Design review of the part built by this model. Coordinates are the model's own, in mm. A direction names the side the tool comes from. Coordinates: 2 decimals unless noted, no trailing zeros. Loops run counter-clockwise (first coordinate to the right, second up) from the corner with the lowest first, then second, coordinate; pieces in that order, holes last. Notation, with made-up numbers: (38, -27.75) - (78, -27.75) arc R31 ccw to (78, 2.25) - close; hole circle Ø3 at (-33, -33). An arc over 180 degrees is marked (long way). Return JSON: item names as keys, results as strings. Group by question number.
from build123d import *

# Parameters (mm, degrees)
SKETCH1_R           = 2.1
SKETCH1_R_2         = 1.6
SKETCH1_W           = 120
SKETCH1_H           = 56
SKETCH1_R_3         = 2.5
SKETCH1_R_4         = 3
BOSS_EXTRUDE1_DEPTH = 7
FILLET1_R           = 6


with BuildPart() as part:
    # Sketch1 → Boss-Extrude1 (new body)
    with BuildSketch(Plane(origin=(0, 0, 0), x_dir=(1, 0, 0), z_dir=(0, 1, 0))):
        Polygon((-125.817930688, 74), (-60, -40), (60, -40), (125.817930688, 74), (7.5, 142.310889132), (5, 137.980762114), (-5, 137.980762114), (-7.5, 142.310889132), align=None)
        with Locations(Location((-69.15767665, -4.138438763, 0), (0, 0, 270))):
            Circle(SKETCH1_R, mode=Mode.SUBTRACT)
        with Locations(Location((-40, -34, 0), (0, 0, 270))):
            Circle(SKETCH1_R, mode=Mode.SUBTRACT)
        with Locations(Location((-88.15767665, 28.770526581, 0), (0, 0, 270))):
            Circle(SKETCH1_R, mode=Mode.SUBTRACT)
        with Locations(Location((-20, 33, 0), (0, 0, 270))):
            Circle(SKETCH1_R_2, mode=Mode.SUBTRACT)
        with Locations(Location((0, -34, 0), (0, 0, 270))):
            Circle(SKETCH1_R, mode=Mode.SUBTRACT)
        with Locations(Location((40, -34, 0), (0, 0, 270))):
            Circle(SKETCH1_R, mode=Mode.SUBTRACT)
        Rectangle(SKETCH1_W, SKETCH1_H, mode=Mode.SUBTRACT)
        with Locations(Location((69.15767665, -4.138438763, 0), (0, 0, 270))):
            Circle(SKETCH1_R, mode=Mode.SUBTRACT)
        with Locations(Location((20, 33, 0), (0, 0, 270))):
            Circle(SKETCH1_R_2, mode=Mode.SUBTRACT)
        with Locations(Location((88.15767665, 28.770526581, 0), (0, 0, 270))):
            Circle(SKETCH1_R, mode=Mode.SUBTRACT)
        with Locations(Location((-107.15767665, 61.679491924, 0), (0, 0, 270))):
            Circle(SKETCH1_R, mode=Mode.SUBTRACT)
        Polygon((-102.72391992, 74), (-101.817930688, 74), (-102.497422612, 73.607695155), align=None, mode=Mode.SUBTRACT)
        with Locations(Location((-20, 53, 0), (0, 0, 270))):
            Circle(SKETCH1_R_2, mode=Mode.SUBTRACT)
        with Locations(Location((-20, 73, 0), (0, 0, 270))):
            Circle(SKETCH1_R_3, mode=Mode.SUBTRACT)
        with Locations(Location((-20, 93, 0), (0, 0, 270))):
            Circle(SKETCH1_R_3, mode=Mode.SUBTRACT)
        with Locations(Location((-10, 107.980762114, 0), (0, 0, 270))):
            Circle(SKETCH1_R_4, mode=Mode.SUBTRACT)
        with Locations(Location((-10, 127.980762114, 0), (0, 0, 270))):
            Circle(SKETCH1_R, mode=Mode.SUBTRACT)
        with Locations(Location((20, 53, 0), (0, 0, 270))):
            Circle(SKETCH1_R_2, mode=Mode.SUBTRACT)
        with Locations(Location((20, 73, 0), (0, 0, 270))):
            Circle(SKETCH1_R_3, mode=Mode.SUBTRACT)
        with Locations(Location((0, 73, 0), (0, 0, 270))):
            Circle(SKETCH1_R_3, mode=Mode.SUBTRACT)
        with Locations(Location((107.15767665, 61.679491924, 0), (0, 0, 270))):
            Circle(SKETCH1_R, mode=Mode.SUBTRACT)
        Polygon((102.497422612, 73.607695155), (101.817930688, 74), (102.72391992, 74), align=None, mode=Mode.SUBTRACT)
        with BuildLine():
            ThreePointArc((2.5, 93), (0, 90.5), (-2.5, 93))
            ThreePointArc((-2.5, 93), (0, 95.5), (2.5, 93))
        make_face(mode=Mode.SUBTRACT)
        with BuildLine():
            ThreePointArc((20, 90.5), (18.232233047, 91.232233047), (17.5, 93))
            ThreePointArc((17.5, 93), (21.767766953, 94.767766953), (20, 90.5))
        make_face(mode=Mode.SUBTRACT)
        with Locations(Location((10, 107.980762114, 0), (0, 0, 270))):
            Circle(SKETCH1_R_4, mode=Mode.SUBTRACT)
        with Locations(Location((10, 127.980762114, 0), (0, 0, 270))):
            Circle(SKETCH1_R, mode=Mode.SUBTRACT)
    extrude(amount=BOSS_EXTRUDE1_DEPTH)

    # Fillet1
    fillet1_edges = [part.edges().sort_by_distance(p)[0] for p in [
        (-60, 3.5, 28),
        (60, 3.5, 28),
        (60, 3.5, 40),
        (-60, 3.5, 40),
    ]]
    fillet(fillet1_edges, radius=FILLET1_R)


solid = part.part
Item 1: For P1, Ø6.5, axis at x = -20, z = -93, coming from the +Y side; P2, Ø4, axis at y = 6, z = -25.5, coming from the +X side, all flat-tipped, find the tip position at first contact; note any pin that passes through.
Item 2: Add section B-B (y = 5.5). Give the number of separate pieces and of enclosed holes in the cut face, then the cut area to 3 significant figures.
Item 3: Draft analysis for pull direction Z (two halves, no side actions). For faces 3 (the face through (-65.831, 3.451, -108.634)), 4 (the face through (21.69, 3.45, -74.84)), 5 (the face through (59.498, 3.549, 39.218)), 6 (the face through (-2, 7, -52)), state which applies: pulls with the +Z half, pulls with the -Z half, needs draft (parallel to the pull), parting line crosses it, or undercut.
Item 4: Add section C-C (z = -41). State the section outline as (x, y) points.
Item 5: Add section A-A (z = -14.5). State the section outline as (x, y) points, then the cut area to 3 significant figures.
Item 6: To check wall thickness, follow line 1 (X direction, y = 4, z = -53); line 2 (X direction, y = 4, z = -33); line 3 (Z direction, x = 45.5, y = 5.5). State the ranges of each line that lie inside material, in increasing order. Write a range as from..to.
Item 7: For faces 1 (the face through (-2, 0, -52)), 2 (the face through (-1, 3, 28)), list the 3-axis set-ups (+Z, -Z, +X, -X, +Y, -Y) from which the entire face can be reached by the end or side of a thin tool; tool diameter is ignored.
Answers below:
{
 "1": {"P1": "stops at y = 7", "P2": "stops at x = 98.97"},
 "2": {"separate pieces": "1", "enclosed holes": "26", "area": "23,200 mm^2"},
 "3": {"face 3": "pulls with the -Z half", "face 4": "undercut", "face 5": "pulls with the +Z half", "face 6": "needs draft"},
 "4": {"outline": "(-106.77, 0) - (106.77, 0) - (106.77, 7) - (-106.77, 7) - close"},
 "5": {"outline": "(-91.47, 0) - (-60, 0) - (-60, 7) - (-91.47, 7) - close; (60, 0) - (91.47, 0) - (91.47, 7) - (60, 7) - close", "area": "441 mm^2"},
 "6": {"line 1": "x = -113.69..-21.6, -18.4..18.4, 21.6..113.69", "line 2": "x = -102.15..-21.6, -18.4..18.4, 21.6..102.15", "line 3": "z = -120.37..-28, 28..40"},
 "7": {"face 1": "+Z, -Z, +X, -X, -Y", "face 2": "+Y, -Y"}
}
